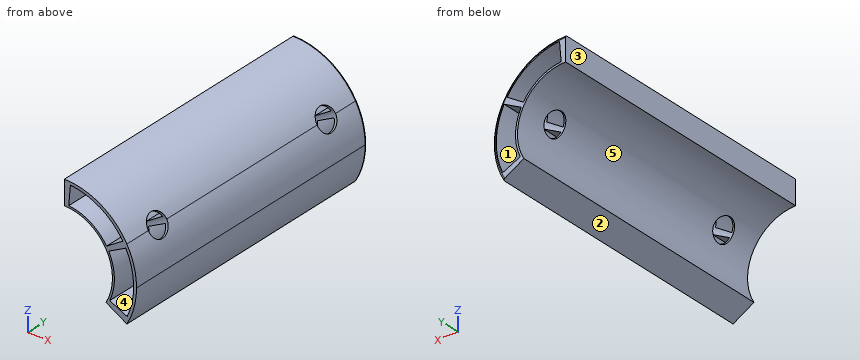
```python
from build123d import *

# Parameters (mm, degrees)
F1_DEPTH = 75
F5_D     = 12
F7_DEPTH = 150
F8_R     = 1


with BuildPart() as f1:
    # F0 (on Front) → F1 (new body, symmetric)
    with BuildSketch(Plane.XZ):
        with BuildLine():
            Line((21.6506350946, 12.5), (32.4759526419, 18.75))
            ThreePointArc((32.4759526419, 18.75), (18.75, 32.4759526419), (0, 37.5))
            Line((0, 37.5), (0, 25))
            ThreePointArc((0, 25), (12.5, 21.6506350946), (21.6506350946, 12.5))
        make_face()
        with BuildLine():
            ThreePointArc((32.4759526419, -18.75), (36.2222184858, -9.7057141913), (37.5, 0))
            ThreePointArc((37.5, 0), (36.2222184858, 9.7057141913), (32.4759526419, 18.75))
            Line((32.4759526419, 18.75), (21.6506350946, 12.5))
            ThreePointArc((21.6506350946, 12.5), (24.1481456572, 6.4704761276), (25, 0))
            ThreePointArc((25, 0), (24.1481456572, -6.4704761276), (21.6506350946, -12.5))
            Line((21.6506350946, -12.5), (32.4759526419, -18.75))
        make_face()
    extrude(amount=F1_DEPTH, both=True)

    # F5 (through all)
    with Locations(Plane(origin=(33.5584843966, 0, 19.375), x_dir=(0, -1, 0), z_dir=(0.8660254038, 0, 0.5))):
        with Locations((55, 0), (-55, 0)):
            Hole(F5_D / 2)

    # F6 (on face) → F7 (cut)
    with BuildSketch(Plane(origin=(0, 75, 0), x_dir=(-1, 0, 0), z_dir=(0, 1, 0))):
        with BuildLine():
            ThreePointArc((-21.9281775911, 13.969789817), (-13.4881047122, 22.2277086375), (-2.2660493114, 25.9010621504))
            Line((-2.2660493114, 25.9010621504), (-3.1376067389, 35.8630091313))
            ThreePointArc((-3.1376067389, 35.8630091313), (-18.6758372938, 30.7768273442), (-30.3620920493, 19.3427859005))
            Line((-30.3620920493, 19.3427859005), (-21.9281775911, 13.969789817))
        make_face()
        with BuildLine():
            ThreePointArc((-23.564002463, -10.9880748053), (-25.9938127041, 0.5671870109), (-23.0622816626, 12.0054639441))
            Line((-23.0622816626, 12.0054639441), (-31.9323899944, 16.6229500765))
            ThreePointArc((-31.9323899944, 16.6229500765), (-35.9914329749, 0.7853358612), (-32.6270803333, -15.2142574227))
            Line((-32.6270803333, -15.2142574227), (-23.564002463, -10.9880748053))
        make_face()
    extrude(amount=-F7_DEPTH, mode=Mode.SUBTRACT)

    # F8
    f8_edges = [f1.edges().sort_by_distance(p)[0] for p in [
        (32.475953, 75, 18.75),
    ]]
    fillet(f8_edges, radius=F8_R)


solid = f1.part
```
Read the model definition and answer for the solid it produces. Units are mm, in the model's axes. Face numbers are marked on the shaded views. A direction names the side the tool comes from. Coordinates: 2 decimals unless noted, no trailing zeros. Order: outer loops, then holes, each group sorted by start corner. A loop starts at its lowest first (then second) coordinate and runs counter-clockwise, first axis right, second up. Notation, with made-up numbers: (-14, -13) - (29, -13) arc R20 ccw to (29, 12) - close; hole circle Ø6 at (52.5, 48.25). An arc over 180 degrees is marked (long way). Answer as a JSON object with one key per item and string values. Group by question number.
Item 1: Flat-ended cylindrical pins translate along their axes: P1, Ø1, axis at x = 29.5, y = 10.5, coming from the -Z side; P2, Ø5, axis at x = 31.5, z = 6.5, coming from the +Y side; P3, Ø12, axis at x = 20, y = 55.5, coming from the -Z side; P4, Ø10, axis at y = 27, z = 14, coming from the -X side. Find the tip coordinate at first contact, or state that the pin passes through.
Item 2: Consider probe 1 along X at (y, z) = (44, 1); probe 2 along X at (y, z) = (-15.5, -14); probe 3 along Z at (x, y) = (28, -68). Determine where each line is inside the solid, lowest interval first. Write a range as from..to.
Item 3: A tool of negligible diameter and unlimited length cuts with its end or side. For the marked faces 4 and 5, from which of +Z, -Z, +X, -X, +Y, -Y can it reach the whole face along a straight path? Write none if from no direction.
Item 4: The mould has two halves that part along Z. Classify the marked faces 1, 2 and 3: +Z half, -Z half, draft (parallel to the pull), parting line (faces both ways), or undercut.
Item 5: Section B-B (y = 57) is taken. Give the vertices of the cut face in (x, z).
Item 6: Section A-A (y = 9.5) is taken. Give the vertices of the cut face in (x, z).
Results are:
{
 "1": {"P1": "stops at z = -17.32", "P2": "passes through", "P3": "stops at z = -15.01", "P4": "stops at x = 16.25"},
 "2": {"probe 1": "x = 24.98..25.98, 35.99..37.49", "probe 2": "x = 24.25..30.02, 33.17..34.79", "probe 3": "z = -16.17..-13.06, 14.58..17.84, 22.63..24.94"},
 "3": {"face 4": "+Y, -Y", "face 5": "-X, +Y, -Y"},
 "4": {"face 1": "undercut", "face 2": "-Z half", "face 3": "draft"},
 "5": {"outline": "(0, 25) arc R25 cw to (18.26, 17.07) - (19.15, 17.59) arc R26 ccw to (2.27, 25.9) - (3.14, 35.86) arc R36 cw to (27.96, 22.68) - (29.28, 23.43) arc R37.5 ccw to (0, 37.5) - close; (21.65, -12.5) - (32.48, -18.75) arc R37.5 ccw to (34.93, 13.64) - (33.62, 12.88) arc R36 cw to (32.63, -15.21) - (23.56, -10.99) arc R26 ccw to (24.81, 7.79) - (23.92, 7.28) arc R25 cw to start"},
 "6": {"outline": "(0, 25) arc R25 cw to (21.65, -12.5) - (32.48, -18.75) arc R37.5 ccw to (0, 37.5) - close; hole (2.27, 25.9) arc R26 cw to (21.93, 13.97) - (30.36, 19.34) arc R36 ccw to (3.14, 35.86) - close; hole (23.06, 12.01) arc R26 cw to (23.56, -10.99) - (32.63, -15.21) arc R36 ccw to (31.93, 16.62) - close"}
}
